Autodesk Inventor part; units mm, degrees
ref_plane "YZ Plane" through (0, 0, 0) normal (1, 0, 0) x (0, 1, 0)
ref_plane "XZ Plane" through (0, 0, 0) normal (0, 1, 0) x (-1, 0, 0)
ref_plane "XY Plane" through (0, 0, 0) normal (0, 0, 1) x (1, 0, 0)
sketch "Sketch1" plane through (0, 0, 0) normal (0, 1, 0) x (-1, 0, 0)
  line L0 (31.575, 38.95) -> (-5.625, 38.95)
  line L1 (-5.625, 38.95) -> (-33.925, -36.6)
  line L2 (-33.925, -36.6) -> (-28.075, -42.45)
  line L3 (-28.075, -42.45) -> (28.075, -42.45)
  line L4 (28.075, -42.45) -> (31.575, -38.95)
  line L5 (31.575, -38.95) -> (31.575, 38.95)
  point P0 (0, 0)
  point P1 (0, -42.45)
  point P2 (31.575, 0)
  dimension "d0" = 3.5
  dimension "d1" = 3.5
  dimension "d2" = 81.4
  dimension "d3" = 37.2
  dimension "d4" = 65.5
  dimension "d5" = 59.65
extrude "Extrusion1" add sketch "Sketch1" along normal mid plane 13.7
equation "\"d1\" = d0"
properties part number "StrategyCard_All" material "Paper"
Geometry check sheet. Reference: the model listing, model coordinates, mm. Give positions to 0.01 mm unless a question says otherwise; leave off trailing zeros. Loops run counter-clockwise (first coordinate to the right, second up) from the corner with the lowest first, then second, coordinate; pieces in that order, holes last. Notation, with made-up numbers: M 53,-2.5 L 72,-2.5 A20 cw 72,31.5 Z; hole C -11.5,13 d8. An arc over 180 degrees is marked long. Write item = value, one per line. Start each with the question number.
1. Section check C-C, the plane x = 15.5. Enter the section's corners in (y, z), plus the area to 3 significant figures.
2. Section check A-A, the plane y = 0. Enter the section's corners in (x, z) (3 decimals).
3. Thickness scan on probe 1 along X at (y, z) = (6.25, 3) (3 decimals); probe 2 along X at (y, z) = (4, 32) (3 decimals). Record the ranges inside material, lowest first.
4. Section check B-B, the plane z = -19. Enter the section's corners in (x, y) (3 decimals).
5. Go/stop test with flat-tipped pins: P1, Ø4, axis at y = -4, z = 11.5, coming from the +X side; P2, Ø8, axis at x = 13, z = 22.5, coming from the +Y side. Record where each tip stops, or that it passes through.
Values follow:
q1.outline = M -6.85,-42.45 L 6.85,-42.45 L 6.85,12.59 L -6.85,12.59 Z
q1.area = 754 mm^2
q2.outline = M -31.575,-38.95 L -28.075,-42.45 L 28.075,-42.45 L 33.925,-36.6 L 5.625,38.95 L -31.575,38.95 Z
q3.probe_1 = -31.575 to 19.091
q3.probe_2 = -31.575 to 8.228
q4.outline = M -31.575,-6.85 L 27.332,-6.85 L 27.332,6.85 L -31.575,6.85 Z
q5.P1 = 16.66
q5.P2 = 6.85
